```python
from build123d import *

# Parameters (mm, degrees)
BOSS_EXTRUDE1_DEPTH = 2
CUT_EXTRUDE1_DEPTH  = 0.5
SKETCH3_R           = 1
CUT_EXTRUDE2_DEPTH  = 2.5


with BuildPart() as part:
    # Sketch1 → Boss-Extrude1 (new body)
    with BuildSketch(Plane(origin=(0, 0, 0), x_dir=(0, 0, -1), z_dir=(1, 0, 0))):
        with BuildLine():
            Line((0, 0), (0, 6.5))
            ThreePointArc((0, 6.5), (4, 10.5), (8, 6.5))
            Line((8, 6.5), (8, 0))
            Line((8, 0), (0, 0))
        make_face()
    extrude(amount=BOSS_EXTRUDE1_DEPTH)

    # Sketch2 → Cut-Extrude1 (cut)
    with BuildSketch(Plane.ZY):
        with BuildLine():
            Line((-8, 3), (-6, 3))
            Line((-6, 3), (-6, 0))
            Line((-6, 0), (-2, 0))
            Line((-2, 0), (-2, 3))
            Line((-2, 3), (0, 3))
            Line((0, 3), (0, 6.5))
            ThreePointArc((0, 6.5), (-4, 10.5), (-8, 6.5))
            Line((-8, 6.5), (-8, 3))
        make_face()
    extrude(amount=-CUT_EXTRUDE1_DEPTH, mode=Mode.SUBTRACT)

    # Sketch3 → Cut-Extrude2 (cut, through all)
    with BuildSketch(Plane.ZY.offset(-0.5)):
        with Locations((-4, 6)):
            Circle(SKETCH3_R)
    extrude(amount=-CUT_EXTRUDE2_DEPTH, mode=Mode.SUBTRACT)


solid = part.part
```
Input: part model. Units: mm. Frame: model coordinates. Round coordinates to 2 decimals unless told otherwise and drop trailing zeros. Loops run counter-clockwise (first coordinate to the right, second up) from the corner with the lowest first, then second, coordinate; pieces in that order, holes last. Notation, with made-up numbers: (21, -7) -> (72, -7) arc R12 ccw to (72, 10) -> close; hole circle Ø2 at (-35.75, 24.5). An arc over 180 degrees is marked (long way). Use one line per item in the form item = value. Start each with the question number.
Item 1: Contact query for flat-ended pins moving along their axis: pin 1 Ø0.6 at (x, z) = (0, -0.5) entering from +Y; pin 2 Ø3 at (y, z) = (6, -4) entering from -X; pin 3 Ø0.6 at (x, y) = (0, 2) entering from +Z. Output: stop coordinate, or through.
Item 2: Mould query, pull axis Y, two halves, no side actions, for faces 1 (the face through (1.2, 10.5, -3.9)), 2 (the face through (1.24, 6.676, -4.737)), 3 (the face through (0, 2, -1)), 4 (the face through (1, 0, -4)). Classes: pulls with the +Y half, pulls with the -Y half, needs draft (parallel to the pull), parting line crosses it, or undercut.
Item 3: Material intervals for L1, parallel to Y at x = 1, z = -4; L2, parallel to X at y = 3.75, z = -2.25; L3, parallel to Z at x = 0.1, y = 0.75, sorted ascending. Write a range as from..to.
Item 4: Section query D-D on y = 3.25. Return the cut outline in (x, z), then the cut area to 3 significant figures.
Item 5: Section query C-C on x = 1.75. Return the cut outline in (y, z).
Item 6: Section query B-B on z = -4. Return the cut outline in (x, y), then the cut area to 4 significant figures.
Item 7: Section query A-A on y = 6. Return the cut outline in (x, z), then the cut area to 3 significant figures.
Ans:
q1.pin_1 = 3
q1.pin_2 = 0.5
q1.pin_3 = 0
q2.face_1 = pulls with the +Y half
q2.face_2 = undercut
q2.face_3 = needs draft
q2.face_4 = pulls with the -Y half
q3.L1 = 0..5, 7..10.5
q3.L2 = 0.5..2
q3.L3 = -8..-6, -2..0
q4.outline = (0.5, -8) -> (2, -8) -> (2, 0) -> (0.5, 0) -> close
q4.area = 12.0 mm^2
q5.outline = (0, -8) -> (6.5, -8) arc R4 ccw to (6.5, 0) -> (0, 0) -> close; hole circle Ø2 at (6, -4)
q6.outline = (0.5, 0) -> (2, 0) -> (2, 5) -> (0.5, 5) -> close; (0.5, 7) -> (2, 7) -> (2, 10.5) -> (0.5, 10.5) -> close
q6.area = 12.75 mm^2
q7.outline = (0.5, -8) -> (2, -8) -> (2, -5) -> (0.5, -5) -> close; (0.5, -3) -> (2, -3) -> (2, 0) -> (0.5, 0) -> close
q7.area = 9.00 mm^2
